from build123d import *

# Parameters (mm, degrees)
SKETCH_R     = 1
PAD_DEPTH    = 6
POCKET_DEPTH = 5


with BuildPart() as part:
    # Sketch → Pad (new body)
    with BuildSketch(Plane.XY):
        with BuildLine():
            ThreePointArc((4.5, 9.5), (0, 14), (-4.5, 9.5))
            Line((-4.5, 9.5), (-4.5, -9.5))
            ThreePointArc((-4.5, -9.5), (0, -14), (4.5, -9.5))
            Line((4.5, -9.5), (4.5, 9.5))
        make_face()
        with Locations((0, 9.5)):
            Circle(SKETCH_R, mode=Mode.SUBTRACT)
        with Locations((0, -9.5)):
            Circle(SKETCH_R, mode=Mode.SUBTRACT)
    extrude(amount=PAD_DEPTH)

    # Sketch001 (on Face8 of Pad) → Pocket (cut)
    with BuildSketch(Plane.XY.offset(6)):
        with BuildLine():
            ThreePointArc((3.5, 9.5), (0, 13), (-3.5, 9.5))
            Line((-3.5, 9.5), (-2, -4))
            ThreePointArc((-2, -4), (0, -6), (2, -4))
            Line((3.5, 9.5), (2, -4))
        make_face()
    extrude(amount=-POCKET_DEPTH, mode=Mode.SUBTRACT)


solid = part.part
Read the model definition and answer for the solid it produces. Units are mm, in the model's axes. A direction names the side the tool comes from. Give positions to 0.01 mm unless a question says otherwise; leave off trailing zeros. Write each loop counter-clockwise with the first axis right and the second up, starting at its lowest first coordinate (ties: lowest second). Pieces come first, ordered by that corner, then holes. Notation, with made-up numbers: (63.25, 28) - (102.25, 28) arc R26 cw to (102.25, 46) - close; hole circle Ø8 at (34.25, 13.25). An arc over 180 degrees is marked (long way). Answer in a Markdown table with one row per item. Add a question column.
Item 1: Find the intervals of material crossed by L1, parallel to Y at x = 0, z = 0.3; L2, parallel to Y at x = 0, z = 3.45; L3, parallel to X at y = 9.5, z = 0.5, in increasing order.
Item 2: Determine the mould class of faces 3 (the face through (0, -14, 3)), 4 (the face through (0, 4, 1)), 5 (the face through (4.5, 0, 3)) for opening direction X: pulls with the +X half, pulls with the -X half, needs draft (parallel to the pull), parting line crosses it, or undercut.
Item 3: Section C-C, the plane y = -4.5 is taken. Write down the section's boundary in (x, z), and give its area (3 significant figures).
Item 4: Section B-B, the plane x = 0 is taken. Write down the section's boundary in (y, z), and give its area (3 significant figures).
Item 5: Flat-ended cylindrical pins translate along their axes: P1, Ø3, axis at x = 2.5, z = 4.5, coming from the +Y side; P2, Ø2, axis at x = -2.5, z = 4.5, coming from the +Y side; P3, Ø1.5, axis at x = -1, z = 4, coming from the +Y side. Find the tip coordinate at first contact, or state that the pin passes through.
Item 6: A tool of negligible diameter and unlimited length cuts with its end or side. For faces 1 (the face through (0, 13, 4)), 2 (the face through (0, 0, 0)), from which of +Z, -Z, +X, -X, +Y, -Y can it reach the whole face along a straight path? Write none if from no direction.
Item 7: Section A-A, the plane z = 5.6 is taken. Write down the section's boundary in (x, y), and give its area (3 significant figures).
Item 8: Section D-D, the plane x = 1.5 is taken. Write down the section's boundary in (y, z).
Recorded:
| question | item | result |
|---|---|---|
| 1 | L1 | y = -14 to -10.5, -8.5 to 8.5, 10.5 to 14 |
| 1 | L2 | y = -14 to -10.5, -8.5 to -6, 13 to 14 |
| 1 | L3 | x = -4.5 to -1, 1 to 4.5 |
| 2 | face 3 | parting line crosses it |
| 2 | face 4 | undercut |
| 2 | face 5 | pulls with the +X half |
| 3 | outline | (-4.5, 0) - (4.5, 0) - (4.5, 6) - (1.94, 6) - (1.94, 1) - (-1.94, 1) - (-1.94, 6) - (-4.5, 6) - close |
| 3 | area | 34.6 mm2 |
| 4 | outline | (-14, 0) - (-10.5, 0) - (-10.5, 6) - (-14, 6) - close; (-8.5, 0) - (8.5, 0) - (8.5, 1) - (-6, 1) - (-6, 6) - (-8.5, 6) - close; (10.5, 0) - (14, 0) - (14, 6) - (13, 6) - (13, 1) - (10.5, 1) - close |
| 4 | area | 59.0 mm2 |
| 5 | P1 | stops at y = 13.89 |
| 5 | P2 | stops at y = 13.74 |
| 5 | P3 | stops at y = 13.99 |
| 6 | face 1 | +Z |
| 6 | face 2 | -Z, +X, -X, +Y, -Y |
| 7 | outline | (-4.5, -9.5) arc R4.5 ccw to (4.5, -9.5) - (4.5, 9.5) arc R4.5 ccw to (-4.5, 9.5) - close; hole (-3.5, 9.5) - (-2, -4) arc R2 ccw to (2, -4) - (3.5, 9.5) arc R3.5 ccw to start; hole circle Ø2 at (0, -9.5) |
| 7 | area | 132 mm2 |
| 8 | outline | (-13.74, 0) - (13.74, 0) - (13.74, 6) - (12.66, 6) - (12.66, 1) - (-5.32, 1) - (-5.32, 6) - (-13.74, 6) - close |
